```python
from build123d import *

# Parameters (mm, degrees)
SKETCH1_W              = 35
SKETCH1_H              = 20
BASE_PLATE_DEPTH       = 3
SKETCH2_W              = 35
SKETCH2_H              = 5
SIDE_WALLS_DEPTH       = 18
SKETCH4_R              = 1.5
SKETCH4_R_2            = 1.25
M2_SCREWS_DEPTH        = 18
SKETCH6_W              = 5
SKETCH6_H              = 20
RETURN_STOPPER_DEPTH   = 4.5
SKETCH9_W              = 12
SKETCH9_H              = 16
BOSS_EXTRUDE1_DEPTH    = 4.5
SKETCH7_R              = 7.75
MAGNET_POCKET_DEPTH    = 6
SKETCH8_R              = 2
M2_SCREW_HEAD_DEPTH    = 1.5
M3_ACHSLE_DEPTH        = 36.429507476
M3_ACHSLE_DEPTH_BACK   = 36.429507476
SKETCH5_R              = 1.625
SKETCH14_R             = 3.5
CUT_EXTRUDE1_DEPTH     = 1.5
CUT_EXTRUDE2_START     = -1.5
SKETCH15_R             = 3.5
CUT_EXTRUDE2_DEPTH     = 1.5
FILLET1_R              = 1.5
LEAVER_START           = -0.25
SKETCH11_W             = 22
SKETCH11_H             = 10.5
LEAVER_SPACE_DEPTH     = 20.5
SKETCH12_W             = 17
SKETCH12_H             = 4.5
MORE_SPACE_LEFT_DEPTH  = 0.25
SKETCH13_W             = 17
SKETCH13_H             = 4.5
MORE_SPACE_RIGHT_DEPTH = 0.25
FILLET2_R              = 0.75
FILLET3_R              = 0.75
FILLET4_R              = 0.75
FILLET5_R              = 0.5
CHAMFER1_SIZE          = 3.5
CHAMFER1_SIZE_2        = 9.616170968


with BuildPart() as part:
    # Sketch1 → Base Plate (new body)
    with BuildSketch(Plane.XY):
        Rectangle(SKETCH1_W, SKETCH1_H)
    extrude(amount=BASE_PLATE_DEPTH)

    # Sketch2 → Side Walls (add)
    with BuildSketch(Plane(origin=(0, 0, 0), x_dir=(1, 0, 0), z_dir=(0, 0, -1))):
        with Locations((0, -12.5)):
            Rectangle(SKETCH2_W, SKETCH2_H)
        with Locations((0, 12.5)):
            Rectangle(SKETCH2_W, SKETCH2_H)
    extrude(amount=-SIDE_WALLS_DEPTH)

    # Sketch4 → M2 Screws (cut)
    with BuildSketch(Plane.XY.offset(18)):
        with Locations((-14.5, -12.5)):
            Circle(SKETCH4_R)
        with Locations((7.5, -12.5)):
            Circle(SKETCH4_R)
        with Locations((7.5, 12.5)):
            Circle(SKETCH4_R_2)
        with Locations((-14.5, 12.5)):
            Circle(SKETCH4_R_2)
    extrude(amount=-M2_SCREWS_DEPTH, mode=Mode.SUBTRACT)

    # Sketch6 → Return Stopper (add)
    with BuildSketch(Plane.XY.offset(3)):
        with Locations((15, 0)):
            Rectangle(SKETCH6_W, SKETCH6_H)
    extrude(amount=RETURN_STOPPER_DEPTH)

    # Sketch9 → Boss-Extrude1 (add)
    with BuildSketch(Plane.XY.offset(3)):
        with Locations((6.5, 0)):
            Rectangle(SKETCH9_W, SKETCH9_H)
    extrude(amount=BOSS_EXTRUDE1_DEPTH)

    # Sketch7 → Magnet Pocket (cut)
    with BuildSketch(Plane(origin=(0, 0, 0), x_dir=(-1, 0, 0), z_dir=(0, 0, 1))):
        with Locations(Location((-8.75, 0, 0), (0, 0, 90))):
            Circle(SKETCH7_R)
    extrude(amount=MAGNET_POCKET_DEPTH, mode=Mode.SUBTRACT)

    # Sketch8 → M2 Screw Head (cut)
    with BuildSketch(Plane(origin=(0, 0, 0), x_dir=(1, 0, 0), z_dir=(0, 0, -1))):
        with Locations(Location((7.5, -12.5, 0), (0, 0, 270))):
            Circle(SKETCH8_R)
        with Locations(Location((-14.5, -12.5, 0), (0, 0, 270))):
            Circle(SKETCH8_R)
        with Locations(Location((7.5, 12.5, 0), (0, 0, 270))):
            Circle(SKETCH8_R)
        with Locations(Location((-14.5, 12.5, 0), (0, 0, 270))):
            Circle(SKETCH8_R)
    extrude(amount=-M2_SCREW_HEAD_DEPTH, mode=Mode.SUBTRACT)

    # Sketch5 → M3 Achsle (cut, two sides: drawn at the far end of the back side and taken through both)
    with BuildSketch(Plane.XZ.offset(-10).offset(-M3_ACHSLE_DEPTH_BACK)):
        with Locations((-10.5, 11)):
            Circle(SKETCH5_R)
    extrude(amount=M3_ACHSLE_DEPTH + M3_ACHSLE_DEPTH_BACK, mode=Mode.SUBTRACT)

    # Sketch14 → Cut-Extrude1 (cut)
    with BuildSketch(Plane(origin=(0, 15, 0), x_dir=(-1, 0, 0), z_dir=(0, 1, 0))):
        with Locations((10.5, 11)):
            Circle(SKETCH14_R)
    extrude(amount=-CUT_EXTRUDE1_DEPTH, mode=Mode.SUBTRACT)

    # Sketch15 → Cut-Extrude2 (cut)
    with BuildSketch(Plane.XZ.offset(15).offset(CUT_EXTRUDE2_START)):
        with Locations(Location((-10.5, 11, 0), (0, 0, 180))):
            Circle(SKETCH15_R)
    extrude(amount=CUT_EXTRUDE2_DEPTH, mode=Mode.SUBTRACT)

    # Fillet1
    fillet1_edges = [part.edges().sort_by_distance(p)[0] for p in [
        (0.5, 0, 7.5),
    ]]
    fillet(fillet1_edges, radius=FILLET1_R)

    # Sketch11 → Leaver Space (cut)
    with BuildSketch(Plane.XZ.offset(-10).offset(LEAVER_START)):
        with Locations((6.5, 12.75)):
            Rectangle(SKETCH11_W, SKETCH11_H)
    extrude(amount=LEAVER_SPACE_DEPTH, mode=Mode.SUBTRACT)

    # Sketch12 → More Space left (cut)
    with BuildSketch(Plane.XZ.offset(-10)):
        with Locations((4, 5.25)):
            Rectangle(SKETCH12_W, SKETCH12_H)
    extrude(amount=-MORE_SPACE_LEFT_DEPTH, mode=Mode.SUBTRACT)

    # Sketch13 → More Space right (cut)
    with BuildSketch(Plane(origin=(0, -10, 0), x_dir=(-1, 0, 0), z_dir=(0, 1, 0))):
        with Locations((-4, 5.25)):
            Rectangle(SKETCH13_W, SKETCH13_H)
    extrude(amount=-MORE_SPACE_RIGHT_DEPTH, mode=Mode.SUBTRACT)

    # Fillet2
    # the kernel refuses this fillet: 0.75 mm, written as the material it takes off along each edge
    with BuildSketch(Plane(origin=(19.375, 15, 0), x_dir=(0, -1, 0), z_dir=(-1, 0, 0))) as fillet2_piece_1:
        with BuildLine():
            CenterArc((FILLET2_R, FILLET2_R), FILLET2_R, 180, 90)
            Line((0, FILLET2_R), (0, 0))
            Line((0, 0), (FILLET2_R, 0))
        make_face()
    extrude(amount=38.75, mode=Mode.SUBTRACT)

    # Fillet3
    # the kernel refuses this fillet: 0.75 mm, written as the material it takes off along each edge
    with BuildSketch(Plane(origin=(-19.375, -15, 0), x_dir=(0, 1, 0), z_dir=(1, 0, 0))) as fillet3_piece_1:
        with BuildLine():
            CenterArc((FILLET3_R, FILLET3_R), FILLET3_R, 180, 90)
            Line((0, FILLET3_R), (0, 0))
            Line((0, 0), (FILLET3_R, 0))
        make_face()
    extrude(amount=38.75, mode=Mode.SUBTRACT)

    # Fillet4
    fillet4_edges = [part.edges().sort_by_distance(p)[0] for p in [
        (-17.5, -15, 9.375),
        (-17.5, 0, 0),
        (-17.5, 14.780330086, 0.219669914),
        (-17.5, -14.780330086, 0.219669914),
        (-17.5, 15, 9.375),
    ]]
    fillet(fillet4_edges, radius=FILLET4_R)

    # Fillet5
    fillet5_edges = [part.edges().sort_by_distance(p)[0] for p in [
        (17.5, -15, 9.375),
        (17.5, 14.780330086, 0.219669914),
        (17.5, 0, 0),
        (17.5, -14.780330086, 0.219669914),
        (17.5, 15, 9.375),
    ]]
    fillet(fillet5_edges, radius=FILLET5_R)

    # Chamfer1
    # the kernel refuses this chamfer: 9.616170968, 3.5 mm, written as the material it takes off along each edge
    with BuildSketch(Plane(origin=(17.5, -14.696220073, 18), x_dir=(-0.9950833631817486, 0, 0.09904090225205049), z_dir=(0, 1, 0))) as chamfer1_piece_1:
        Polygon((CHAMFER1_SIZE * 0.995083363182, -CHAMFER1_SIZE * 0.0990409022521), (-CHAMFER1_SIZE_2 * 0.099040902253, -CHAMFER1_SIZE_2 * 0.995083363191), (0, 0), align=None)
    extrude(amount=54.142440145, mode=Mode.SUBTRACT)
    with BuildSketch(Plane(origin=(17.5, -39.446220073, 18), x_dir=(0.013184058198645607, 0, -0.9999130865277316), z_dir=(0, 1, 0))) as chamfer1_piece_2:
        Polygon((CHAMFER1_SIZE_2 * 0.999913086537, CHAMFER1_SIZE_2 * 0.0131840581988), (-CHAMFER1_SIZE * 0.0131840581986, CHAMFER1_SIZE * 0.999913086528), (0, 0), align=None)
    extrude(amount=54.142440145, mode=Mode.SUBTRACT)


solid = part.part
```
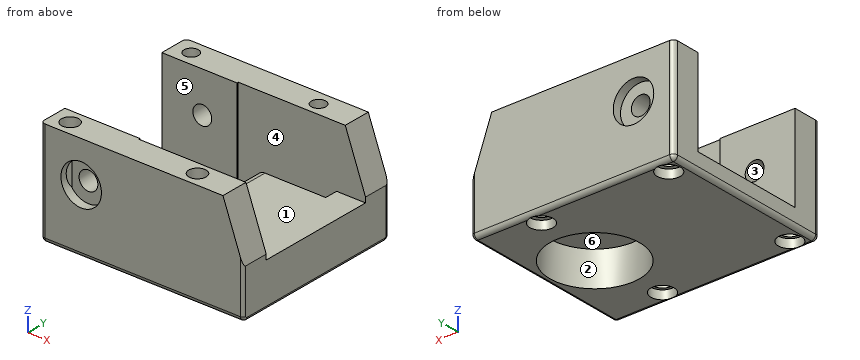
Check sheet for the modelled part. Datum: model origin and axes. Units: mm. Face numbers are marked on the shaded views. A direction names the side the tool comes from. Give positions to 0.01 mm unless a question says otherwise; leave off trailing zeros. Loops run counter-clockwise (first coordinate to the right, second up) from the corner with the lowest first, then second, coordinate; pieces in that order, holes last. Notation, with made-up numbers: M 39.25,-4 L 61.25,-4 A31 ccw 61.25,33 Z; hole C -14.75,46 d10. An arc over 180 degrees is marked long. Answer as CSV lines item,"result".
Item 1: Sectioned sample at D-D, the plane x = -6. Enter the section's corners in (y, z).
Reply:
outline,"M -15,0.75 A0.75 ccw -14.25,0 L 14.25,0 A0.75 ccw 15,0.75 L 15,18 L 10,18 L 10,3 L -10,3 L -10,18 L -15,18 Z"
Item 2: Depth check by flat-ended pin: pin 1 Ø2.5 at (x, y) = (7.5, -12.5) entering from +Z; pin 2 Ø8 at (x, y) = (6.5, -2) entering from +Z; pin 3 Ø5.5 at (x, z) = (-10.5, 11) entering from +Y; pin 4 Ø0.9 at (y, z) = (1, 5) entering from -X. Enter the tip coordinate at first touch or a pass-through.
Reply:
pin 1,"through"
pin 2,"z = 7.5"
pin 3,"y = 13.5"
pin 4,"x = 0.5"
Item 3: Draft check along Z on the marked faces 1, 2 and 3. Enter one of: pulls with the +Z half, pulls with the -Z half, needs draft (parallel to the pull), parting line crosses it, or undercut.
Reply:
face 1,"pulls with the +Z half"
face 2,"needs draft"
face 3,"undercut"
Item 4: Sectioned sample at B-B, the plane x = -10.5. Enter the section's corners in (y, z) (3 decimals), then the cut area to 3 significant figures.
Reply:
outline,"M -15,0.75 A0.75 ccw -14.25,0 L 14.25,0 A0.75 ccw 15,0.75 L 15,7.5 L 13.5,7.5 L 13.5,9.375 L 10,9.375 L 10,3 L -10,3 L -10,9.375 L -13.5,9.375 L -13.5,7.5 L -15,7.5 Z; M -15,14.5 L -13.5,14.5 L -13.5,12.625 L -10,12.625 L -10,18 L -15,18 Z; M 10,12.625 L 13.5,12.625 L 13.5,14.5 L 15,14.5 L 15,18 L 10,18 Z"
area,"196 mm^2"
Item 5: Sectioned sample at A-A, the plane y = 12.5. Enter the section's corners in (x, z) (3 decimals).
Reply:
outline,"M -17.5,0.75 A0.75 ccw -16.75,0 L -16.5,0 L -16.5,1.5 L -15.75,1.5 L -15.75,18 L -17.5,18 Z; M -13.25,1.5 L -12.5,1.5 L -12.5,0 L 5.5,0 L 5.5,1.5 L 6.25,1.5 L 6.25,18 L -13.25,18 Z; M 8.75,1.5 L 9.5,1.5 L 9.5,0 L 17,0 A0.5 ccw 17.5,0.5 L 17.5,8.384 L 14,18 L 8.75,18 Z; hole C -10.5,11 d3.25"
Item 6: Sectioned sample at C-C, the plane z = 11. State how many separate pieces and enclosed holes the cut face has, then the cut area to 3 significant figures.
Reply:
separate pieces,"4"
enclosed holes,"2"
area,"262 mm^2"
Item 7: Set-up check for the marked faces 4, 5 and 6: record each of +Z, -Z, +X, -X, +Y, -Y from which the full face is reachable in a straight line by a thin tool's end or side.
Reply:
face 4,"+Z"
face 5,"+Z, -X"
face 6,"-Z"
Item 8: Scan lines: L1, parallel to X at y = -12.5, z = 1.15; L2, parallel to Y at x = -14.5, z = 13.5; L3, parallel to Y at x = -14.5, z = 1. Record each from-to range of solid material in increasing order.
Reply:
L1,"-17.5 to -16.5, -12.5 to 5.5, 9.5 to 17.5"
L2,"-15 to -14, -11 to -10, 10 to 11.25, 13.75 to 15"
L3,"-15 to -14.5, -10.5 to 10.5, 14.5 to 15"
